Check sheet for the modelled part. Datum: model origin and axes. Units: mm. A direction names the side the tool comes from. Coordinates: 2 decimals unless noted, no trailing zeros. Loops run counter-clockwise (first coordinate to the right, second up) from the corner with the lowest first, then second, coordinate; pieces in that order, holes last.
from build123d import *

# Parameters (mm, degrees)
F0_R          = 3
F0_R_2        = 2.5
F1_DEPTH      = 180.504
F2_R          = 2
F3_R          = 7
F6_DEPTH      = 30
F6_DEPTH_BACK = 30


# Not quite as in the source:
# - a feature names something its author has since deleted; it is built from what else it names


with BuildPart() as f1:
    # F0 (on Top) → F1 (new body)
    with BuildSketch(Plane.XY):
        with BuildLine():
            Line((18.15, -30), (30, -30))
            Line((30, -30), (30, -18.15))
            Line((30, -18.15), (27.5, -18.15))
            Line((27.5, -18.15), (27.5, -20.15))
            Line((27.5, -20.15), (21.5477069044, -20.15))
            ThreePointArc((21.5477069044, -20.15), (19.5, -15), (21.5477069044, -9.85))
            Line((21.5477069044, -9.85), (27.5, -9.85))
            Line((27.5, -9.85), (27.5, -11.85))
            Line((27.5, -11.85), (30, -11.85))
            Line((30, -11.85), (30, 11.85))
            Line((30, 11.85), (27.5, 11.85))
            Line((27.5, 11.85), (27.5, 9.85))
            Line((27.5, 9.85), (21.5477069044, 9.85))
            ThreePointArc((21.5477069044, 9.85), (19.5, 15), (21.5477069044, 20.15))
            Line((21.5477069044, 20.15), (27.5, 20.15))
            Line((27.5, 20.15), (27.5, 18.15))
            Line((27.5, 18.15), (30, 18.15))
            Line((30, 18.15), (30, 30))
            Line((30, 30), (18.15, 30))
            Line((18.15, 30), (18.15, 27.5))
            Line((18.15, 27.5), (20.15, 27.5))
            Line((20.15, 27.5), (20.15, 21.5477069044))
            ThreePointArc((20.15, 21.5477069044), (15, 19.5), (9.85, 21.5477069044))
            Line((9.85, 21.5477069044), (9.85, 27.5))
            Line((9.85, 27.5), (11.85, 27.5))
            Line((11.85, 27.5), (11.85, 30))
            Line((11.85, 30), (-11.85, 30))
            Line((-11.85, 30), (-11.85, 27.5))
            Line((-11.85, 27.5), (-9.85, 27.5))
            Line((-9.85, 27.5), (-9.85, 21.5477069044))
            ThreePointArc((-9.85, 21.5477069044), (-15, 19.5), (-20.15, 21.5477069044))
            Line((-20.15, 21.5477069044), (-20.15, 27.5))
            Line((-20.15, 27.5), (-18.15, 27.5))
            Line((-18.15, 27.5), (-18.15, 30))
            Line((-18.15, 30), (-30, 30))
            Line((-30, 30), (-30, 18.15))
            Line((-30, 18.15), (-27.5, 18.15))
            Line((-27.5, 18.15), (-27.5, 20.15))
            Line((-27.5, 20.15), (-21.5477069044, 20.15))
            ThreePointArc((-21.5477069044, 20.15), (-19.5, 15), (-21.5477069044, 9.85))
            Line((-21.5477069044, 9.85), (-27.5, 9.85))
            Line((-27.5, 9.85), (-27.5, 11.85))
            Line((-27.5, 11.85), (-30, 11.85))
            Line((-30, 11.85), (-30, -11.85))
            Line((-30, -11.85), (-27.5, -11.85))
            Line((-27.5, -11.85), (-27.5, -9.85))
            Line((-27.5, -9.85), (-21.5477069044, -9.85))
            ThreePointArc((-21.5477069044, -9.85), (-19.5, -15), (-21.5477069044, -20.15))
            Line((-21.5477069044, -20.15), (-27.5, -20.15))
            Line((-27.5, -20.15), (-27.5, -18.15))
            Line((-27.5, -18.15), (-30, -18.15))
            Line((-30, -18.15), (-30, -30))
            Line((-30, -30), (-18.15, -30))
            Line((-18.15, -30), (-18.15, -27.5))
            Line((-18.15, -27.5), (-20.15, -27.5))
            Line((-20.15, -27.5), (-20.15, -21.5477069044))
            ThreePointArc((-20.15, -21.5477069044), (-15, -19.5), (-9.85, -21.5477069044))
            Line((-9.85, -21.5477069044), (-9.85, -27.5))
            Line((-9.85, -27.5), (-11.85, -27.5))
            Line((-11.85, -27.5), (-11.85, -30))
            Line((-11.85, -30), (11.85, -30))
            Line((11.85, -30), (11.85, -27.5))
            Line((11.85, -27.5), (9.85, -27.5))
            Line((9.85, -27.5), (9.85, -21.5477069044))
            ThreePointArc((9.85, -21.5477069044), (15, -19.5), (20.15, -21.5477069044))
            Line((20.15, -21.5477069044), (20.15, -27.5))
            Line((20.15, -27.5), (18.15, -27.5))
            Line((18.15, -27.5), (18.15, -30))
        make_face()
        with Locations((-25, -25)):
            Circle(F0_R, mode=Mode.SUBTRACT)
        with Locations((-15, -15)):
            Circle(F0_R_2, mode=Mode.SUBTRACT)
        with Locations((25, -25)):
            Circle(F0_R, mode=Mode.SUBTRACT)
        with Locations((15, -15)):
            Circle(F0_R_2, mode=Mode.SUBTRACT)
        with Locations((-25, 25)):
            Circle(F0_R, mode=Mode.SUBTRACT)
        with Locations((-15, 15)):
            Circle(F0_R_2, mode=Mode.SUBTRACT)
        Polygon((-7, 22), (-7, 27.5), (0, 27.5), (7, 27.5), (7, 22), (10, 16), (10, 10), (16, 10), (22, 7), (27.5, 7), (27.5, 0), (27.5, -7), (22, -7), (16, -10), (10, -10), (10, -16), (7, -22), (7, -27.5), (0, -27.5), (-7, -27.5), (-7, -22), (-10, -16), (-10, -10), (-16, -10), (-22, -7), (-27.5, -7), (-27.5, 0), (-27.5, 7), (-22, 7), (-16, 10), (-10, 10), (-10, 16), align=None, mode=Mode.SUBTRACT)
        with Locations((15, 15)):
            Circle(F0_R_2, mode=Mode.SUBTRACT)
        with Locations((25, 25)):
            Circle(F0_R, mode=Mode.SUBTRACT)
    extrude(amount=F1_DEPTH)

    # F2
    f2_edges = [f1.edges().sort_by_distance(p)[0] for p in [
        (-7, 27.5, 90.252),
        (7, 27.5, 90.252),
    ]]
    fillet(f2_edges, radius=F2_R)

    # F3
    f3_edges = [f1.edges().sort_by_distance(p)[0] for p in [
        (-10, 16, 90.252),
        (10, 16, 90.252),
    ]]
    fillet(f3_edges, radius=F3_R)

    # F5 (on Right) → F6 (cut, two sides)
    with BuildSketch(Plane.YZ) as f6_sk:
        Polygon((166.5976946582, -66.7170951811), (146.3493769552, 35.0780720561), (-30, 0), (-9.751682297, -101.7951672372), align=None)
        Polygon((135.5963626007, 147.5648354856), (151.7094622056, 228.5708574701), (-13.8869003951, 261.5100219845), (-30, 180.504), align=None)
    extrude(amount=F6_DEPTH, mode=Mode.SUBTRACT)
    extrude(f6_sk.sketch, amount=-F6_DEPTH_BACK, mode=Mode.SUBTRACT)


solid = f1.part
(1) Section check A-A, the plane x = 25. Enter the section's corners in (y, z), plus the area to 3 significant figures.
(2) Scan lines: line 1 along Y through (x, z) = (25, 95); line 2 along Y through (x, z) = (15, 61). Record each from-to range of solid material in increasing order.
(3) Draft check along X on faces 1 (the face through (24, 30, 89)), 2 (the face through (8.5, -19, 89)), 3 (the face through (30, -24, 89)). Enter one of: pulls with the +X half, pulls with the -X half, needs draft (parallel to the pull), parting line crosses it, or undercut.
(4) Set-up check for faces 4 (the face through (19, 8.5, 89.1)), 5 (the face through (0, -30, 89)): record each of +Z, -Z, +X, -X, +Y, -Y from which the full face is reachable in a straight line by a thin tool's end or side.
(5) Section check B-B, the plane y = -25. Enter the section's corners in (x, z).
(6) Gauge pin test, flat ends, axial feed: P1, Ø1.5, axis at x = -16.5, z = 136.5, coming from the +Y side; P2, Ø3, axis at x = -15, y = 15, coming from the +Z side. Record the tip position at first contact, or that the pin passes through.
(7) Section check C-C, the plane z = 124.5. Count the separate pieces of the cut face and the enclosed holes in it, plus the area to 3 significant figures.
Determined:
1. outline: (-30, 0) - (-28, 0.4) - (-28, 180.11) - (-30, 180.5) - close; (-22, 1.59) - (-20.15, 1.96) - (-20.15, 178.54) - (-22, 178.91) - close; (-9.85, 4.01) - (-7, 4.57) - (-7, 175.93) - (-9.85, 176.5) - close; (7, 7.36) - (9.85, 7.93) - (9.85, 172.58) - (7, 173.14) - close; (20.15, 9.98) - (22, 10.34) - (22, 170.16) - (20.15, 170.53) - close; (28, 11.54) - (30, 11.93) - (30, 168.57) - (28, 168.97) - close
1. area: 2,260 mm2
2. line 1: y = -30 to -28, -22 to -20.15, -9.85 to -7, 7 to 9.85, 20.15 to 22, 28 to 30
2. line 2: y = -19.5 to -17.5, -12.5 to -10, 10 to 12.5, 17.5 to 19.5
3. face 1: needs draft
3. face 2: undercut
3. face 3: pulls with the +X half
4. face 4: +Z, -Z
4. face 5: +Z, -Z, +X, -X, -Y
5. outline: (-30, 0.99) - (-28, 0.99) - (-28, 179.51) - (-30, 179.51) - close; (-22, 0.99) - (-20.15, 0.99) - (-20.15, 179.51) - (-22, 179.51) - close; (-9.85, 0.99) - (-7, 0.99) - (-7, 179.51) - (-9.85, 179.51) - close; (7, 0.99) - (9.85, 0.99) - (9.85, 179.51) - (7, 179.51) - close; (20.15, 0.99) - (22, 0.99) - (22, 179.51) - (20.15, 179.51) - close; (28, 0.99) - (30, 0.99) - (30, 179.51) - (28, 179.51) - close
6. P1: stops at y = 19.85
6. P2: passes through
7. separate pieces: 1
7. enclosed holes: 9
7. area: 1,080 mm2
